Check sheet for the modelled part. Datum: model origin and axes. Units: mm. Round coordinates to 2 decimals unless told otherwise and drop trailing zeros. Write each loop counter-clockwise with the first axis right and the second up, starting at its lowest first coordinate (ties: lowest second). Pieces come first, ordered by that corner, then holes. Notation, with made-up numbers: (45.25, 0) - (81.25, 0) arc R17 ccw to (81.25, 31) - close; hole circle Ø8 at (-10.75, 56). An arc over 180 degrees is marked (long way). Answer as a JSON object with one key per item and string values. Group by question number.
Item 1: Sectioned sample at A-A on y = -220. Record the boundary of the cut face in (x, z).
Item 2: Sectioned sample at D-D on z = 857.5. Record the boundary of the cut face in (x, y), plus the area to 3 significant figures.
Item 3: Sectioned sample at B-B on z = 115. Record the boundary of the cut face in (x, y).
Item 4: Gauge pin test, flat ends, axial feed: P1, Ø20, axis at x = -597, y = -204.5, coming from the -Z side; P2, Ø12, axis at x = 600, y = -53.5, coming from the +Z side. Record the tip position at first contact, or that the pin passes through.
Item 5: Thickness scan on line 1 (X direction, y = -148.5, z = -32). Record the ranges inside material, lowest first.
Item 6: Sectioned sample at C-C on x = -500. Record the boundary of the cut face in (y, z), plus the area to 3 significant figures.
```python
from build123d import *

# Parameters (mm, degrees)
F0_W          = 40
F0_H          = 40
F1_DEPTH      = 760
F1_DEPTH_BACK = 145
F2_W          = 1150
F2_H          = 40
F2_W_2        = 40
F2_H_2        = 565
F2_H_3        = 5
F3_DEPTH      = 40
F0_W_2        = 1150
F0_H_2        = 570
F4_DEPTH      = 40
F2_H_4        = 35
F5_DEPTH      = 240
F6_W          = 40
F6_H          = 40
F7_DEPTH      = 200
F8_W          = 40
F8_H          = 40
F9_DEPTH      = 200


with BuildPart() as f1:
    # F0 (on Top) → F1 (new body, two sides)
    with BuildSketch(Plane.XY) as f1_sk:
        with Locations((595, 305)):
            Rectangle(F0_W, F0_H)
    extrude(amount=F1_DEPTH)
    extrude(f1_sk.sketch, amount=-F1_DEPTH_BACK)



with BuildPart() as f1b:
    # F0 (on Top) → F1, piece 2 (new body, two sides)
    with BuildSketch(Plane.XY) as f1_2_sk:
        with Locations((-595, 305)):
            Rectangle(F0_W, F0_H)
    extrude(amount=F1_DEPTH)
    extrude(f1_2_sk.sketch, amount=-F1_DEPTH_BACK)


with BuildPart() as f1c:
    # F0 (on Top) → F1, piece 3 (new body, two sides)
    with BuildSketch(Plane.XY) as f1_3_sk:
        with Locations((-595, -305)):
            Rectangle(F0_W, F0_H)
    extrude(amount=F1_DEPTH)
    extrude(f1_3_sk.sketch, amount=-F1_DEPTH_BACK)


with BuildPart() as f1d:
    # F0 (on Top) → F1, piece 4 (new body, two sides)
    with BuildSketch(Plane.XY) as f1_4_sk:
        with Locations((595, -305)):
            Rectangle(F0_W, F0_H)
    extrude(amount=F1_DEPTH)
    extrude(f1_4_sk.sketch, amount=-F1_DEPTH_BACK)


with BuildPart() as f1_1:
    add(f1.part)

    add(f1b.part)  # F3 merges F1b

    add(f1c.part)  # F3 merges F1c

    add(f1d.part)  # F3 merges F1d
    # F2 (on face) → F3 (join)
    with BuildSketch(Plane.XY.offset(760)):
        with Locations((0, 305)):
            Rectangle(F2_W, F2_H)
        with Locations((595, 2.5)):
            Rectangle(F2_W_2, F2_H_2)
        Polygon((-575, -325), (575, -325), (575, -320), (575, -285), (-575, -285), (-575, -320), align=None)
        with Locations((-595, 2.5)):
            Rectangle(F2_W_2, F2_H_2)
        with Locations((-595, -282.5)):
            Rectangle(F2_W_2, F2_H_3)
        with Locations((595, -282.5)):
            Rectangle(F2_W_2, F2_H_3)
    extrude(amount=-F3_DEPTH)

    # F0 (on Top) → F4 (join)
    with BuildSketch(Plane.XY):
        with Locations((0, -305)):
            Rectangle(F0_W_2, F0_H)
        with Locations((595, 0)):
            Rectangle(F0_W, F0_H_2)
        with Locations((0, 305)):
            Rectangle(F0_W_2, F0_H)
        with Locations((-595, 0)):
            Rectangle(F0_W, F0_H_2)
    extrude(amount=-F4_DEPTH)

    # F2 (on face) → F5 (join)
    with BuildSketch(Plane.XY.offset(760)):
        with Locations((-595, -302.5)):
            Rectangle(F2_W_2, F2_H_4)
        with Locations((-595, -282.5)):
            Rectangle(F2_W_2, F2_H_3)
        with Locations((595, -302.5)):
            Rectangle(F2_W_2, F2_H_4)
        with Locations((595, -282.5)):
            Rectangle(F2_W_2, F2_H_3)
    extrude(amount=F5_DEPTH)

    # F6 (on face) → F7 (join)
    with BuildSketch(Plane(origin=(0, -280, 0), x_dir=(-1, 0, 0), z_dir=(0, 1, 0))):
        with Locations((-595, 980)):
            Rectangle(F6_W, F6_H)
    extrude(amount=F7_DEPTH)

    # F8 (on face) → F9 (join)
    with BuildSketch(Plane(origin=(0, -280, 0), x_dir=(-1, 0, 0), z_dir=(0, 1, 0))):
        with Locations((595, 980)):
            Rectangle(F8_W, F8_H)
    extrude(amount=F9_DEPTH)


solid = f1_1.part
```
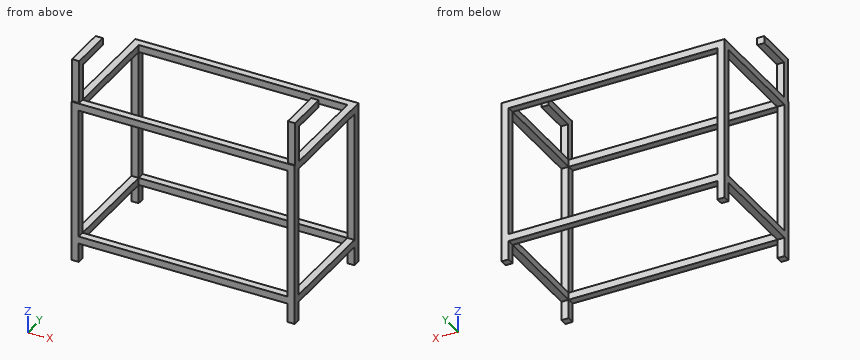
Completed:
{
 "1": {"outline": "(-615, -40) - (-575, -40) - (-575, 0) - (-615, 0) - close; (-615, 720) - (-575, 720) - (-575, 760) - (-615, 760) - close; (-615, 960) - (-575, 960) - (-575, 1000) - (-615, 1000) - close; (575, -40) - (615, -40) - (615, 0) - (575, 0) - close; (575, 720) - (615, 720) - (615, 760) - (575, 760) - close; (575, 960) - (615, 960) - (615, 1000) - (575, 1000) - close"},
 "2": {"outline": "(-615, -320) - (-575, -320) - (-575, -280) - (-615, -280) - close; (575, -320) - (615, -320) - (615, -280) - (575, -280) - close", "area": "3,200 mm²"},
 "3": {"outline": "(-615, -325) - (-575, -325) - (-575, -285) - (-615, -285) - close; (-615, 285) - (-575, 285) - (-575, 325) - (-615, 325) - close; (575, -325) - (615, -325) - (615, -285) - (575, -285) - close; (575, 285) - (615, 285) - (615, 325) - (575, 325) - close"},
 "4": {"P1": "z = -40", "P2": "z = 760"},
 "5": {"line 1": "-615 to -575, 575 to 615"},
 "6": {"outline": "(-325, -40) - (-285, -40) - (-285, 0) - (-325, 0) - close; (-325, 720) - (-285, 720) - (-285, 760) - (-325, 760) - close; (285, -40) - (325, -40) - (325, 0) - (285, 0) - close; (285, 720) - (325, 720) - (325, 760) - (285, 760) - close", "area": "6,400 mm²"}
}
